The listing builds one solid part. Answer for the finished solid, in the listing's coordinates (mm). Face numbers are marked on the shaded views. Give positions to 0.01 mm unless a question says otherwise; leave off trailing zeros. Answer as a JSON object with one key per item and string values. Group by question number.
Q1. Consider line 1 (Y direction, x = -24.35, z = 1.5); line 2 (X direction, y = -11.5, z = 9.75); line 3 (X direction, y = -12.65, z = 1.5). Determine where each line is inside the solid, lowest interval first.
Q2. The mould has two halves that part along Z. Classify the marked faces 1 and 2: released by +Z, released by -Z, zero draft, split by the parting line, or undercut.
Q3. Given pin 1 (0.5 mm diameter, centred on y = -13.5, z = 1.5, fed in from +X); pin 2 (1 mm diameter, centred on y = -12.5, z = 3, fed in from -X); pin 3 (0.7 mm diameter, centred on y = -12.5, z = 1, fed in from -X), each flat-ended and moving along its own axis, determine where each tip first touches the part or whether it passes through.
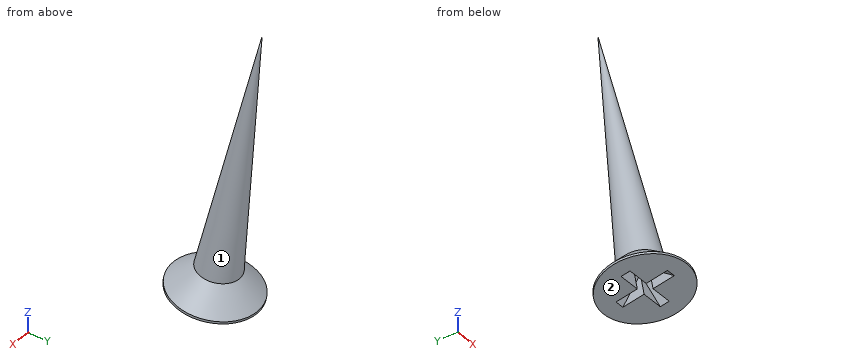
from build123d import *

# Parameters (mm, degrees)
POCKET004_DEPTH         = 0.2
POLARPATTERN001_COUNT   = 2
POLARPATTERN001_ANGLE   = 90
BODY007_ROLL_ANGLE      = -170
BODY007_PLACEMENT_ANGLE = 180


with BuildPart() as part:
    # Sketch022 → Revolution001 (revolve)
    with BuildSketch(Plane.XZ):
        Polygon((0, 0), (0, -12), (0.9, -1.05), (1.85, -0.1), (1.85, 0), align=None)
    revolve(axis=Axis((0, 0, 0), (0, 0, 1)))

    # Sketch023 → Pocket004 (cut, symmetric)
    with BuildSketch(Plane.XZ):
        Polygon((-1.15, 0), (0, -1.15), (1.15, 0), align=None)
    pocket004 = extrude(amount=POCKET004_DEPTH, both=True, mode=Mode.SUBTRACT)

    # PolarPattern001: Pocket004 ×2 about axis
    polarpattern001_axis = Axis((0, 0, 0), (0, 0, 1))
    for i in range(1, POLARPATTERN001_COUNT):
        add(pocket004.rotate(polarpattern001_axis, i * POLARPATTERN001_ANGLE / (POLARPATTERN001_COUNT - 1)), mode=Mode.SUBTRACT)


with BuildPart() as part_1:
    # Body007 roll: moved
    add(part.part.rotate(Axis((0, 0, 0), (1, 0, 0)), BODY007_ROLL_ANGLE))


with BuildPart() as part_2:
    # Body007 placement: moved
    add(part_1.part.moved(Location((-24, -13, 1))).rotate(Axis((-24, -13, 1), (0, 0, 1)), BODY007_PLACEMENT_ANGLE))


solid = part_2.part
Reply:
{
 "1": {"line 1": "y = -14.65 to -13.11, -12.71 to -11.71", "line 2": "x = -24.25 to -23.75", "line 3": "x = -25.37 to -24.2, -23.8 to -22.63"},
 "2": {"face 1": "undercut", "face 2": "released by -Z"},
 "3": {"pin 1": "stops at x = -22.29", "pin 2": "stops at x = -24.86", "pin 3": "stops at x = -25.84"}
}
